```python
from build123d import *

# Parameters (mm, degrees)
SKETCH1_W                     = 279.6
SKETCH1_H                     = 216.6
BOSS_EXTRUDE1_DEPTH           = 2.5
SKETCH2_W                     = 222.6
SKETCH2_H                     = 285.6
SKETCH2_W_2                   = 216.6
SKETCH2_H_2                   = 279.6
BOSS_EXTRUDE2_WALL_30MM_DEPTH = 30
BOSS_EXTRUDE3_DEPTH           = 20
CHAMFER1_SIZE                 = 1


with BuildPart() as part:
    # Sketch1 → Boss-Extrude1 (new body)
    with BuildSketch(Plane(origin=(0, 0, 0), x_dir=(0, 1, 0), z_dir=(0, 0, 1))):
        Rectangle(SKETCH1_W, SKETCH1_H)
    extrude(amount=BOSS_EXTRUDE1_DEPTH)

    # Sketch2 → Boss-Extrude2 wall 30mm (add)
    with BuildSketch(Plane(origin=(0, 0, 0), x_dir=(1, 0, 0), z_dir=(0, 0, -1))):
        Rectangle(SKETCH2_W, SKETCH2_H)
        Rectangle(SKETCH2_W_2, SKETCH2_H_2, mode=Mode.SUBTRACT)
    extrude(amount=-BOSS_EXTRUDE2_WALL_30MM_DEPTH)

    # Sketch3 → Boss-Extrude3 (add)
    with BuildSketch(Plane.XY.offset(2.5)):
        Polygon((1.5, 71.4), (108.3, 71.4), (108.3, 68.4), (1.5, 68.4), (1.5, 1.5), (108.3, 1.5), (108.3, -1.5), (1.5, -1.5), (1.5, -68.85), (108.3, -68.4), (108.3, -71.4), (1.5, -71.85), (1.5, -139.8), (-1.5, -139.8), (-1.5, -71.85), (-108.3, -71.4), (-108.3, -68.4), (-1.5, -68.85), (-1.5, -1.5), (-108.3, -1.5), (-108.3, 1.5), (-1.5, 1.5), (-1.5, 68.4), (-108.3, 68.4), (-108.3, 71.4), (-1.5, 71.4), (-1.5, 139.8), (1.5, 139.8), align=None)
    extrude(amount=BOSS_EXTRUDE3_DEPTH)

    # Chamfer1
    chamfer1_edges = [part.edges().sort_by_distance(p)[0] for p in [
        (-111.3, -142.8, 15),
        (111.3, -142.8, 15),
        (111.3, 142.8, 15),
        (-111.3, 142.8, 15),
    ]]
    chamfer(chamfer1_edges, length=CHAMFER1_SIZE)


solid = part.part
```
Source: CAD feature listing. Evaluate the final solid. Frame: model axes, mm. Give positions to 0.01 mm unless a question says otherwise; leave off trailing zeros. Loops run counter-clockwise (first coordinate to the right, second up) from the corner with the lowest first, then second, coordinate; pieces in that order, holes last. Notation, with made-up numbers: (2, 89) -> (37, 89) arc R22 ccw to (37, 113) -> close; hole circle Ø4 at (-25, 76.25). An arc over 180 degrees is marked (long way). Use a Markdown table: item, result. Add a question column.
(1) First-contact query: pin 1 Ø20.5 at (x, y) = (32, -113.5) entering from +Z. Flat tip, straight axial feed; report the tip coordinate or a pass-through.
(2) Section query C-C (x = -10). Output: boundary loops of the cut face in (y, z).
(3) Ray query, line 1 (X direction, y = 32, z = 19); line 2 (Y direction, x = 10, z = 6.75); line 3 (Y direction, x = 58, z = 8.5). Return the intervals inside material, ascending.
(4) Pull-direction query (Y, two-part tool) for faces 1 (the face through (-2, -142.8, 15)), 2 (the face through (-56, 105, 2.5)); classes: +Y half, -Y half, draft (parallel to the pull), parting line (faces both ways), or undercut.
(5) Section query A-A (y = -98). Output: boundary loops of the cut face in (x, z).
(6) Section query B-B (z = 27). Output: boundary loops of the cut face in (x, y).
(7) Section query D-D (z = 7.25). Count the separate pieces of the cut face and the enclosed holes in it, then the cut area to 3 significant figures.
Checked values:
| question | item | result |
|---|---|---|
| 1 | pin 1 | z = 2.5 |
| 2 | outline | (-142.8, 0) -> (142.8, 0) -> (142.8, 30) -> (139.8, 30) -> (139.8, 2.5) -> (71.4, 2.5) -> (71.4, 22.5) -> (68.4, 22.5) -> (68.4, 2.5) -> (1.5, 2.5) -> (1.5, 22.5) -> (-1.5, 22.5) -> (-1.5, 2.5) -> (-68.81, 2.5) -> (-68.81, 22.5) -> (-71.81, 22.5) -> (-71.81, 2.5) -> (-139.8, 2.5) -> (-139.8, 30) -> (-142.8, 30) -> close |
| 3 | line 1 | -111.3 to -108.3, -1.5 to 1.5, 108.3 to 111.3 |
| 3 | line 2 | -142.8 to -139.8, -71.81 to -68.81, -1.5 to 1.5, 68.4 to 71.4, 139.8 to 142.8 |
| 3 | line 3 | -142.8 to -139.8, -71.61 to -68.61, -1.5 to 1.5, 68.4 to 71.4, 139.8 to 142.8 |
| 4 | face 1 | -Y half |
| 4 | face 2 | undercut |
| 5 | outline | (-111.3, 0) -> (111.3, 0) -> (111.3, 30) -> (108.3, 30) -> (108.3, 2.5) -> (1.5, 2.5) -> (1.5, 22.5) -> (-1.5, 22.5) -> (-1.5, 2.5) -> (-108.3, 2.5) -> (-108.3, 30) -> (-111.3, 30) -> close |
| 6 | outline | (-111.3, -141.8) -> (-110.3, -142.8) -> (110.3, -142.8) -> (111.3, -141.8) -> (111.3, 141.8) -> (110.3, 142.8) -> (-110.3, 142.8) -> (-111.3, 141.8) -> close; hole (-108.3, -139.8) -> (108.3, -139.8) -> (108.3, 139.8) -> (-108.3, 139.8) -> close |
| 7 | separate pieces | 1 |
| 7 | enclosed holes | 8 |
| 7 | area | 5,770 mm^2 |
